CAD build for the part. Positions are in the model's coordinates, mm. A direction names the side the tool comes from. Round coordinates to 2 decimals unless told otherwise and drop trailing zeros. Loops run counter-clockwise (first coordinate to the right, second up) from the corner with the lowest first, then second, coordinate; pieces in that order, holes last.
```python
from build123d import *

# Parameters (mm, degrees)
SZKIC1_W                    = 190
SZKIC1_H                    = 145
DODANIE_WYCI_GNI_CIE1_DEPTH = 25
SZKIC2_W                    = 171
SZKIC2_H                    = 35
WYTNIJ_WYCI_GNI_CIE1_DEPTH  = 50
SZKIC3_R                    = 11
WYTNIJ_WYCI_GNI_CIE2_DEPTH  = 7
SZKIC4_R                    = 11
WYTNIJ_WYCI_GNI_CIE3_DEPTH  = 7
SZKIC5_R                    = 5
WYTNIJ_WYCI_GNI_CIE4_DEPTH  = 7
SZKIC7_W                    = 25
SZKIC7_H                    = 10
DODANIE_WYCI_GNI_CIE2_DEPTH = 25
SZKIC8_R                    = 2
WYTNIJ_WYCI_GNI_CIE5_DEPTH  = 12
WYTNIJ_WYCI_GNI_CIE6_DEPTH  = 40
SZYK_LINIOWY1_COUNT         = 3
SZYK_LINIOWY1_PITCH         = 45
SFAZOWANIE1_SIZE            = 15


with BuildPart() as part:
    # Szkic1 → Dodanie-wyciągnięcie1 (new body)
    with BuildSketch(Plane(origin=(0, 0, 0), x_dir=(1, 0, 0), z_dir=(0, 1, 0))):
        Rectangle(SZKIC1_W, SZKIC1_H)
    extrude(amount=DODANIE_WYCI_GNI_CIE1_DEPTH)

    # Szkic2 → Wytnij-wyciągnięcie1 (cut)
    with BuildSketch(Plane(origin=(0, 25, 0), x_dir=(1, 0, 0), z_dir=(0, 1, 0))):
        with Locations((0.5, 0)):
            Rectangle(SZKIC2_W, SZKIC2_H)
        with Locations((0, -45)):
            Rectangle(SZKIC2_W, SZKIC2_H)
        with Locations((0, 45)):
            Rectangle(SZKIC2_W, SZKIC2_H)
    extrude(amount=-WYTNIJ_WYCI_GNI_CIE1_DEPTH, mode=Mode.SUBTRACT)

    # Szkic3 → Wytnij-wyciągnięcie2 (cut)
    with BuildSketch(Plane.ZY.offset(-85.5)):
        with Locations((41, 12.5)):
            Circle(SZKIC3_R)
    wytnij_wyci_gni_cie2 = extrude(amount=-WYTNIJ_WYCI_GNI_CIE2_DEPTH, mode=Mode.SUBTRACT)

    # Szkic4 → Wytnij-wyciągnięcie3 (cut)
    with BuildSketch(Plane.ZY.offset(95)):
        with Locations((41, 12.5)):
            Circle(SZKIC4_R)
    wytnij_wyci_gni_cie3 = extrude(amount=-WYTNIJ_WYCI_GNI_CIE3_DEPTH, mode=Mode.SUBTRACT)

    # Szkic5 → Wytnij-wyciągnięcie4 (cut)
    with BuildSketch(Plane.ZY.offset(88)):
        with Locations((41, 12.5)):
            Circle(SZKIC5_R)
    wytnij_wyci_gni_cie4 = extrude(amount=-WYTNIJ_WYCI_GNI_CIE4_DEPTH, mode=Mode.SUBTRACT)

    # Szkic7 → Dodanie-wyciągnięcie2 (add)
    with BuildSketch(Plane(origin=(0, 25, 0), x_dir=(1, 0, 0), z_dir=(0, 1, 0))):
        with Locations((-107.5, -22.5)):
            Rectangle(SZKIC7_W, SZKIC7_H)
        with Locations((-107.5, -59.5)):
            Rectangle(SZKIC7_W, SZKIC7_H)
    dodanie_wyci_gni_cie2 = extrude(amount=-DODANIE_WYCI_GNI_CIE2_DEPTH)

    # Szkic8 → Wytnij-wyciągnięcie5 (cut)
    with BuildSketch(Plane(origin=(0, 25, 0), x_dir=(1, 0, 0), z_dir=(0, 1, 0))):
        with Locations(Location((-114, -59.5, 0), (0, 0, 270))):
            Circle(SZKIC8_R)
        with Locations(Location((-101, -59.5, 0), (0, 0, 270))):
            Circle(SZKIC8_R)
        with Locations(Location((-108, -22.5, 0), (0, 0, 270))):
            Circle(SZKIC8_R)
        with Locations(Location((-95, -22.5, 0), (0, 0, 270))):
            Circle(SZKIC8_R)
    wytnij_wyci_gni_cie5 = extrude(amount=-WYTNIJ_WYCI_GNI_CIE5_DEPTH, mode=Mode.SUBTRACT)

    # Szkic10 → Wytnij-wyciągnięcie6 (cut)
    with BuildSketch(Plane(origin=(0, 25, 0), x_dir=(1, 0, 0), z_dir=(0, 1, 0))):
        with BuildLine():
            Line((-77.55, -69.1), (-77.55, -62.5))
            Line((-77.55, -62.5), (-79.425, -62.5))
            Line((-79.425, -62.5), (-79.425, -64.360545416))
            ThreePointArc((-79.425, -64.360545416), (-80.25, -68.6), (-81.075, -64.360545416))
            Line((-81.075, -64.360545416), (-81.075, -62.5))
            Line((-81.075, -62.5), (-82.95, -62.5))
            Line((-82.95, -62.5), (-82.95, -69.1))
            Line((-82.95, -69.1), (-77.55, -69.1))
        make_face()
        with BuildLine():
            Line((-79.425, -64.360545416), (-79.425, -62.5))
            Line((-79.425, -62.5), (-81.075, -62.5))
            Line((-81.075, -62.5), (-81.075, -64.360545416))
            ThreePointArc((-81.075, -64.360545416), (-80.25, -68.6), (-79.425, -64.360545416))
        make_face()
    wytnij_wyci_gni_cie6 = extrude(amount=-WYTNIJ_WYCI_GNI_CIE6_DEPTH, mode=Mode.SUBTRACT)

    # Szyk liniowy1: Wytnij-wyciągnięcie2, Wytnij-wyciągnięcie3, Wytnij-wyciągnięcie4, Dodanie-wyciągnięcie2, Wytnij-wyciągnięcie5, Wytnij-wyciągnięcie6 ×3
    with Locations(*[(0, 0, -i * SZYK_LINIOWY1_PITCH) for i in range(1, SZYK_LINIOWY1_COUNT)]):
        add(wytnij_wyci_gni_cie2, mode=Mode.SUBTRACT)
        add(wytnij_wyci_gni_cie3, mode=Mode.SUBTRACT)
        add(wytnij_wyci_gni_cie4, mode=Mode.SUBTRACT)
        add(dodanie_wyci_gni_cie2)
        add(wytnij_wyci_gni_cie5, mode=Mode.SUBTRACT)
        add(wytnij_wyci_gni_cie6, mode=Mode.SUBTRACT)

    # Sfazowanie1
    sfazowanie1_edges = [part.edges().sort_by_distance(p)[0] for p in [
        (-120, 0, 59.5),
        (-120, 0, -26.5),
        (-120, 0, -67.5),
        (-120, 0, 18.5),
    ]]
    chamfer(sfazowanie1_edges, length=SFAZOWANIE1_SIZE)


solid = part.part
```
Item 1: Probe line 1 (Z direction, x = 43.5, y = 17); line 2 (Z direction, x = -82, y = 21); line 3 (X direction, y = 21.25, z = 6.5). List the from-to ranges inside material, lowest first.
Answers follow:
line 1: z = -72.5 to -62.5, -27.5 to -17.5, 17.5 to 27.5, 62.5 to 72.5
line 2: z = -72.5 to -62.5, -20.9 to -17.5, 24.1 to 27.5, 69.1 to 72.5
line 3: x = -95 to -85, 86 to 95
Item 2: Two-plate mould, pull along Z, no slides. Class faces 1 (the flat face through (-120, 20, -26)), 2 (the flat face through (-1, 12, 72.5)), 3 (the flat face through (86, 13, 8)), 4 (the cylindrical face through (-99.017, 19.084, 14.24)): released by +Z, released by -Z, zero draft, split by the parting line, or undercut.
Answers follow:
face 1: zero draft
face 2: released by +Z
face 3: undercut
face 4: undercut
Item 3: 3-axis set-ups, long thin cutter, end or side, ignore diameter. For faces 5 (the flat face through (-105, 15, -35.5)), 6 (the flat face through (-88, 7.8, 43.3)), 7 (the flat face through (-77.55, 13, 66)): which of +Z, -Z, +X, -X, +Y, -Y reach the whole face in a straight line?
Answers follow:
face 5: -X, +Y, -Y
face 6: -X
face 7: +Y, -Y
Item 4: Cut at B-B, the plane z = 33. Give the cut face in (x, y), plus the area to 3 significant figures.
Answers follow:
outline: (-95, 0) - (-85.5, 0) - (-85.5, 25) - (-95, 25) - (-95, 20.05) - (-88, 20.05) - (-88, 4.95) - (-95, 4.95) - close; (85.5, 0) - (95, 0) - (95, 25) - (85.5, 25) - (85.5, 20.05) - (92.5, 20.05) - (92.5, 4.95) - (85.5, 4.95) - close
area: 264 mm2
Item 5: Flat gauge pins, fed straight in: P1, Ø11, axis at y = 17.5, z = 46, coming from the -X side; P2, Ø1.2, axis at x = -100, z = 14, coming from the +Y side; P3, Ø8, axis at y = 5, z = 57.5, coming from the -X side. Where does each tip first touch, or does it go through?
Answers follow:
P1: stops at x = -95
P2: stops at y = 13
P3: stops at x = -114
Item 6: Cut at A-A, the plane x = 35. Give the cut face in (y, z).
Answers follow:
outline: (0, -72.5) - (25, -72.5) - (25, -62.5) - (0, -62.5) - close; (0, -27.5) - (25, -27.5) - (25, -17.5) - (0, -17.5) - close; (0, 17.5) - (25, 17.5) - (25, 27.5) - (0, 27.5) - close; (0, 62.5) - (25, 62.5) - (25, 72.5) - (0, 72.5) - close
